Part print with two shaded views. Sizes in mm from the minimum x, y, z corner. A direction names the side the tool comes from. Round coordinates to 2 decimals unless told otherwise and drop trailing zeros. Loops run counter-clockwise (first coordinate to the right, second up) from the corner with the lowest first, then second, coordinate; pieces in that order, holes last. Notation, with made-up numbers: (35, 52.25) -> (45, 52.25) arc R15 ccw to (45, 70.25) -> close; hole circle Ø1 at (62.25, 35). An arc over 180 degrees is marked (long way). Use a Markdown table: item, result. Add a question column.
Item 1: Flat gauge pins, fed straight in: pin 1 (2 mm diameter, centred on y = 57.5, z = 58, fed in from -X); pin 2 (8 mm diameter, centred on x = 100, z = 20, fed in from -Y); pin 3 (9 mm diameter, centred on x = 10, z = 20, fed in from +Y). Where does each tip first touch, or does it go through?
Item 2: Cut at D-D, the plane x = 58.5. List the corners of the cut face in (y, z), plus the area to 3 significant figures.
Item 3: Cut at B-B, the plane z = 60. List the corners of the cut face in (x, y).
Item 4: Two-plate mould, pull along Z, no slides. Class the marked faces 3, 4 and 5: pulls with the +Z half, pulls with the -Z half, needs draft (parallel to the pull), parting line crosses it, or undercut.
Item 5: Cut at C-C, the plane y = 30. List the corners of the cut face in (x, z), plus the area to 3 significant figures.
Item 6: Probe line 1 (X direction, y = 76.25, z = 60); line 2 (Z direction, x = 85, y = 47.5); line 3 (Y direction, x = 55, z = 5.25). List the from-to ranges inside material, lowest first. Write a range as [from, to].
Item 7: Cut at A-A, the plane y = 45. List the corners of the cut face in (x, z).
Item 8: Which spindle directions (+Z, -Z, +X, -X, +Y, -Y) get a long thin tool onto all of the face, cutting with end or side? Do the marked faces 1 and 2. Say none if no direction does.
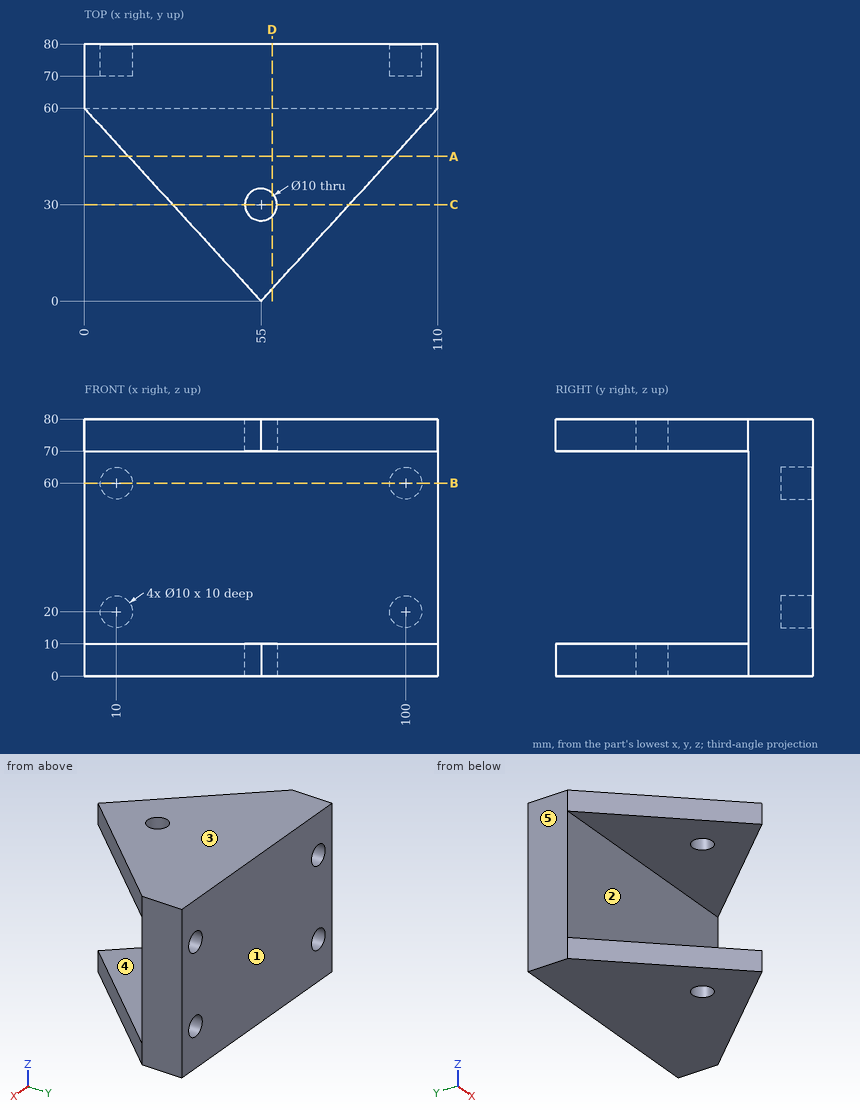
A:
| question | item | result |
|---|---|---|
| 1 | pin 1 | passes through |
| 1 | pin 2 | stops at y = 60 |
| 1 | pin 3 | stops at y = 70 |
| 2 | outline | (3.82, 0) -> (26.43, 0) -> (26.43, 10) -> (3.82, 10) -> close; (3.82, 70) -> (26.43, 70) -> (26.43, 80) -> (3.82, 80) -> close; (33.57, 0) -> (80, 0) -> (80, 80) -> (33.57, 80) -> (33.57, 70) -> (60, 70) -> (60, 10) -> (33.57, 10) -> close |
| 2 | area | 2,580 mm^2 |
| 3 | outline | (0, 60) -> (110, 60) -> (110, 80) -> (105, 80) -> (105, 70) -> (95, 70) -> (95, 80) -> (15, 80) -> (15, 70) -> (5, 70) -> (5, 80) -> (0, 80) -> close |
| 4 | face 3 | pulls with the +Z half |
| 4 | face 4 | undercut |
| 4 | face 5 | needs draft |
| 5 | outline | (27.5, 0) -> (50, 0) -> (50, 10) -> (27.5, 10) -> close; (27.5, 70) -> (50, 70) -> (50, 80) -> (27.5, 80) -> close; (60, 0) -> (82.5, 0) -> (82.5, 10) -> (60, 10) -> close; (60, 70) -> (82.5, 70) -> (82.5, 80) -> (60, 80) -> close |
| 5 | area | 900 mm^2 |
| 6 | line 1 | x = [0, 5], [15, 95], [105, 110] |
| 6 | line 2 | z = [0, 10], [70, 80] |
| 6 | line 3 | y = [0, 25], [35, 80] |
| 7 | outline | (13.75, 0) -> (96.25, 0) -> (96.25, 10) -> (13.75, 10) -> close; (13.75, 70) -> (96.25, 70) -> (96.25, 80) -> (13.75, 80) -> close |
| 8 | face 1 | +Z, -Z, +X, -X, +Y |
| 8 | face 2 | +X, -X, -Y |
